```python
from build123d import *

# Parameters (mm, degrees)
BOSS_EXTRUDE1_DEPTH = 15
FILLET1_R           = 5
SKETCH2_R           = 6
BOSS_EXTRUDE2_DEPTH = 11
SKETCH3_R           = 1.4
BOSS_EXTRUDE3_DEPTH = 65.5
FILLET2_R           = 1


with BuildPart() as part:
    # Sketch1 → Boss-Extrude1 (new body)
    with BuildSketch(Plane(origin=(0, 0, 0), x_dir=(1, 0, 0), z_dir=(0, 1, 0))):
        with BuildLine():
            Line((0, 0), (72, 0))
            ThreePointArc((72, 0), (79.071067812, 2.928932188), (82, 10))
            Line((82, 10), (82, 35))
            ThreePointArc((82, 35), (79.071067812, 42.071067812), (72, 45))
            Line((72, 45), (0, 45))
            Line((0, 45), (0, 0))
        make_face()
    extrude(amount=BOSS_EXTRUDE1_DEPTH)

    # Fillet1
    fillet1_edges = [part.edges().sort_by_distance(p)[0] for p in [
        (79.071067812, 15, -2.928932188),
        (82, 15, -22.5),
        (79.071067812, 15, -42.071067812),
        (36, 15, -45),
        (36, 0, -45),
        (79.071067812, 0, -42.071067812),
        (82, 0, -22.5),
        (79.071067812, 0, -2.928932188),
        (36, 0, 0),
        (36, 15, 0),
    ]]
    fillet(fillet1_edges, radius=FILLET1_R)

    # Sketch2 → Boss-Extrude2 (add, symmetric)
    with BuildSketch(Plane(origin=(82, 0, 0), x_dir=(0, 0, -1), z_dir=(1, 0, 0))):
        with Locations(Location((22.5, 7.5, 0), (0, 0, 155.375681648))):
            Circle(SKETCH2_R)
    extrude(amount=BOSS_EXTRUDE2_DEPTH, both=True)

    # Sketch3 → Boss-Extrude3 (add)
    with BuildSketch(Plane.ZY):
        with Locations(Location((-34.85, 7.5, 0), (0, 0, 180))):
            Circle(SKETCH3_R)
        with Locations(Location((-10.15, 7.5, 0), (0, 0, 180))):
            Circle(SKETCH3_R)
    extrude(amount=BOSS_EXTRUDE3_DEPTH)

    # Fillet2
    fillet2_edges = [part.edges().sort_by_distance(p)[0] for p in [
        (-65.5, 7.5, -33.45),
        (-65.5, 7.5, -8.75),
    ]]
    fillet(fillet2_edges, radius=FILLET2_R)


solid = part.part
```
Could you check a few things on this model? Use its own coordinates, in mm. A direction names the side the tool comes from. Give positions to 0.01 mm unless a question says otherwise; leave off trailing zeros. Loops run counter-clockwise (first coordinate to the right, second up) from the corner with the lowest first, then second, coordinate; pieces in that order, holes last. Notation, with made-up numbers: (-8, -19) -> (14, -19) arc R16 cw to (14, -4) -> close; hole circle Ø2 at (56.25, 79.25). An arc over 180 degrees is marked (long way). Put each result on its own line as item: value.
(1) Imagine slicing it at B-B on z = -22.5. Write out the boundary of the cut face in (x, y), plus the area to 3 significant figures.
Computed:
outline: (0, 0) -> (77, 0) arc R5 ccw to (80.57, 1.5) -> (93, 1.5) -> (93, 13.5) -> (80.57, 13.5) arc R5 ccw to (77, 15) -> (0, 15) -> close
area: 1,350 mm^2
(2) Please list where these lines run through material, in increasing order: probe 1 along X at (y, z) = (6.25, -33.5); probe 2 along X at (y, z) = (9.5, -27.5); probe 3 along Z at (x, y) = (45.5, 2.5). Write a range as [from, to].
Computed:
probe 1: [0, 82]
probe 2: [0, 93]
probe 3: [-44.33, -0.67]
(3) Imagine slicing it at A-A on x = 39. Write out the boundary of the cut face in (y, z), plus the area to 3 significant figures.
Computed:
outline: (0, -40) arc R5 ccw to (5, -45) -> (10, -45) arc R5 ccw to (15, -40) -> (15, -5) arc R5 ccw to (10, 0) -> (5, 0) arc R5 ccw to (0, -5) -> close
area: 654 mm^2
(4) Thinking about a two-plate mould opening in Z: for faces 5 (the face through (37, 7, -45)), 6 (the face through (-31.798, 7.079, -36.185)), 7 (the face through (37, 13, -1)), which applies, pulls with the +Z half, pulls with the -Z half, needs draft (parallel to the pull), parting line crosses it, or undercut?
Computed:
face 5: pulls with the -Z half
face 6: undercut
face 7: pulls with the +Z half
(5) I'm going to push flat-ended pins straight in: pin 1 Ø3 at (y, z) = (2, -15.5) entering from +X; pin 2 Ø1.5 at (y, z) = (7, -12.5) entering from +X; pin 3 Ø3 at (y, z) = (8, -39) entering from +X. Where does each tip first touch, or does it pass through?
Computed:
pin 1: x = 81.77
pin 2: x = 82
pin 3: x = 81.68
(6) For faces 1 (the face through (80, 1, -23)), 2 (the face through (86.87, 1.97, -24.83)), 3 (the face through (80, 14, -23)), 4 (the face through (-31.8, 8.35, -9.04)), which set-ups out of +Z, -Z, +X, -X, +Y, -Y let a thin tool reach every point of the face, with its end or its side?
Computed:
face 1: +X, -Y
face 2: +X
face 3: +X, +Y
face 4: -X
(7) Imagine slicing it at C-C on x = -24. Write out the boundary of the cut face in (y, z), plus the area to 3 significant figures.
Computed:
outline: circle Ø2.8 at (7.5, -34.85); circle Ø2.8 at (7.5, -10.15)
area: 12.3 mm^2
